```python
from build123d import *

# Parameters (mm, degrees)
F0_W     = 203.2
F0_H     = 25.4
F1_DEPTH = 76.2
F3_DEPTH = 25.4
F4_W     = 30.1625
F4_H     = 66.675
F5_DEPTH = 20.6375


with BuildPart() as f1:
    # F0 (on Front) → F1 (new body)
    with BuildSketch(Plane.XZ):
        with Locations((-101.6, 12.7)):
            Rectangle(F0_W, F0_H)
    extrude(amount=F1_DEPTH)

    # F2 (on face) → F3 (cut)
    with BuildSketch(Plane.XY.offset(25.4)):
        with BuildLine():
            Line((0, -76.2), (0, -38.1))
            ThreePointArc((0, -38.1), (-1.8707935661, -57.5073538656), (-7.4142792139, -76.2))
            Line((-7.4142792139, -76.2), (0, -76.2))
        make_face()
        with BuildLine():
            ThreePointArc((-7.4142792139, 0), (-1.8707935661, -18.6926461344), (0, -38.1))
            Line((0, -38.1), (0, 0))
            Line((0, 0), (-7.4142792139, 0))
        make_face()
        with BuildLine():
            ThreePointArc((-195.7857207861, -76.2), (-101.6, -139.7), (-7.4142792139, -76.2))
            Line((-7.4142792139, -76.2), (-195.7857207861, -76.2))
        make_face()
        with BuildLine():
            ThreePointArc((-203.2, -38.1), (-201.3292064339, -18.6926461344), (-195.7857207861, 0))
            Line((-195.7857207861, 0), (-203.2, 0))
            Line((-203.2, 0), (-203.2, -38.1))
        make_face()
        with BuildLine():
            Line((-203.2, -76.2), (-195.7857207861, -76.2))
            ThreePointArc((-195.7857207861, -76.2), (-201.3292064339, -57.5073538656), (-203.2, -38.1))
            Line((-203.2, -38.1), (-203.2, -76.2))
        make_face()
    extrude(amount=-F3_DEPTH, mode=Mode.SUBTRACT)

    # F4 (on face) → F5 (cut)
    with BuildSketch(Plane.XY.offset(25.4)):
        Polygon((-187.325, -4.7625), (-187.325, -38.1), (-187.325, -71.4375), (-136.525, -71.4375), (-136.525, -4.7625), align=None)
        Polygon((-15.875, -71.4375), (-15.875, -38.1), (-15.875, -4.7625), (-66.675, -4.7625), (-66.675, -71.4375), align=None)
        with Locations((-86.51875, -38.1)):
            Rectangle(F4_W, F4_H)
        with Locations((-116.68125, -38.1)):
            Rectangle(F4_W, F4_H)
    extrude(amount=-F5_DEPTH, mode=Mode.SUBTRACT)


solid = f1.part
```
Part model, mm, in its own coordinate system. A direction names the side the tool comes from. Round coordinates to 2 decimals unless told otherwise and drop trailing zeros. Loops run counter-clockwise (first coordinate to the right, second up) from the corner with the lowest first, then second, coordinate; pieces in that order, holes last.
Item 1: Cut at A-A, the plane z = 10.75. Give the cut face in (x, y) (1 decimal).
Item 2: Cut at D-D, the plane z = 1.75. Give the cut face in (x, y).
Item 3: Cut at C-C, the plane y = -20. Give the cut face in (x, z) (1 decimal).
Item 4: Mould opens along X. For faces 1 (the face through (-66.675, -38, 15)), 2 (the face through (-103, -38, 0)), 3 (the face through (-203.2, -38.6, 12.9)) say: +X half, -X half, draft (parallel to the pull), parting line (faces both ways), or undercut.
Item 5: 3-axis set-ups, long thin cutter, end or side, ignore diameter. For faces 4 (the face through (0, -38, 13)), 5 (the face through (-101, -4.763, 15)): which of +Z, -Z, +X, -X, +Y, -Y reach the whole face in a straight line?
Item 6: Cut at B-B, the plane x = -175. Give the cut face in (y, z).
Item 7: Drop flat-ended pins along their axis: P1, Ø1, axis at x = -96.5, y = -12, coming from the +Z side; P2, Ø1, axis at y = -10, z = 11.5, coming from the -X side; P3, Ø3, axis at y = -57, z = 6.5, coming from the -X side. Give the stop position or say it passes through.
Item 8: Drill centre lines: line 1 (X direction, y = -40, z = 6.75) (1 decimal); line 2 (Y direction, x = -174, z = 13); line 3 (X direction, y = -54, z = 14.5) (1 decimal). Where is each one in solid material? Low to high.
A:
1. outline: (-195.8, -76.2) - (-7.4, -76.2) arc R101.6 ccw to (-7.4, 0) - (-195.8, 0) arc R101.6 ccw to start; hole (-187.3, -71.4) - (-136.5, -71.4) - (-136.5, -4.8) - (-187.3, -4.8) - close; hole (-131.8, -71.4) - (-71.4, -71.4) - (-71.4, -4.8) - (-131.8, -4.8) - close; hole (-66.7, -71.4) - (-15.9, -71.4) - (-15.9, -4.8) - (-66.7, -4.8) - close
2. outline: (-195.79, -76.2) - (-7.41, -76.2) arc R101.6 ccw to (-7.41, 0) - (-195.79, 0) arc R101.6 ccw to start
3. outline: (-201.6, 0) - (-1.6, 0) - (-1.6, 25.4) - (-15.9, 25.4) - (-15.9, 4.8) - (-66.7, 4.8) - (-66.7, 25.4) - (-71.4, 25.4) - (-71.4, 4.8) - (-131.8, 4.8) - (-131.8, 25.4) - (-136.5, 25.4) - (-136.5, 4.8) - (-187.3, 4.8) - (-187.3, 25.4) - (-201.6, 25.4) - close
4. face 1: undercut
4. face 2: draft
4. face 3: -X half
5. face 4: +Z, -Z, +X
5. face 5: +Z
6. outline: (-76.2, 0) - (0, 0) - (0, 25.4) - (-4.76, 25.4) - (-4.76, 4.76) - (-71.44, 4.76) - (-71.44, 25.4) - (-76.2, 25.4) - close
7. P1: stops at z = 4.76
7. P2: stops at x = -199.38
7. P3: stops at x = -201.7
8. line 1: x = -203.2 to -187.3, -136.5 to -131.8, -71.4 to -66.7, -15.9 to 0
8. line 2: y = -76.2 to -71.44, -4.76 to 0
8. line 3: x = -201.9 to -187.3, -136.5 to -131.8, -71.4 to -66.7, -15.9 to -1.3
